Verification items for the finished model (mm, model axes). Face numbers are marked on the shaded views. A direction names the side the tool comes from. Coordinates: 2 decimals unless noted, no trailing zeros. Write each loop counter-clockwise with the first axis right and the second up, starting at its lowest first coordinate (ties: lowest second). Pieces come first, ordered by that corner, then holes.
```python
from build123d import *

# Parameters (mm, degrees)
SKETCH1_R           = 6
SKETCH1_R_2         = 1.5
BOSS_EXTRUDE1_DEPTH = 59
SKETCH2_W           = 49
SKETCH2_H           = 46
CUT_EXTRUDE1_DEPTH  = 291.342900723
SKETCH3_W           = 9
SKETCH3_H           = 50
SKETCH3_W_2         = 22
SKETCH3_W_3         = 19
CUT_EXTRUDE2_DEPTH  = 290.584184651
CUT_EXTRUDE3_DEPTH  = 4
SKETCH7_R           = 2.55
CUT_EXTRUDE4_DEPTH  = 82
CUT_EXTRUDE5_DEPTH  = 4
SKETCH9_R           = 1.5
CUT_EXTRUDE6_DEPTH  = 290.584184651


with BuildPart() as part:
    # Sketch1 → Boss-Extrude1 (new body)
    with BuildSketch(Plane(origin=(0, 0, 0), x_dir=(0, 0, -1), z_dir=(1, 0, 0))):
        with BuildLine():
            Line((3, 15), (3, 0))
            Line((3, 0), (283, 0))
            Line((283, 0), (283, 23))
            Line((283, 23), (235, 23))
            Line((235, 23), (235, 10))
            Line((235, 10), (197, 10))
            ThreePointArc((197, 10), (187.807611845, 13.807611845), (184, 23))
            ThreePointArc((184, 23), (180, 27), (176, 23))
            ThreePointArc((176, 23), (172.192388155, 13.807611845), (163, 10))
            Line((163, 10), (32, 10))
            ThreePointArc((32, 10), (28.464466094, 11.464466094), (27, 15))
            ThreePointArc((27, 15), (23.485281374, 23.485281374), (15, 27))
            ThreePointArc((15, 27), (6.514718626, 23.485281374), (3, 15))
        make_face()
        with Locations((15, 15)):
            Circle(SKETCH1_R, mode=Mode.SUBTRACT)
        with Locations((180, 23)):
            Circle(SKETCH1_R_2, mode=Mode.SUBTRACT)
    extrude(amount=BOSS_EXTRUDE1_DEPTH)

    # Sketch2 → Cut-Extrude1 (cut, through all)
    with BuildSketch(Plane.XZ):
        with Locations((24.5, -26)):
            Rectangle(SKETCH2_W, SKETCH2_H)
    extrude(amount=-CUT_EXTRUDE1_DEPTH, mode=Mode.SUBTRACT)

    # Sketch3 → Cut-Extrude2 (cut, through all)
    with BuildSketch(Plane(origin=(0, 10, 0), x_dir=(1, 0, 0), z_dir=(0, 1, 0))):
        with Locations((31, 172)):
            Rectangle(SKETCH3_W, SKETCH3_H)
        with Locations((11, 172)):
            Rectangle(SKETCH3_W_2, SKETCH3_H)
        with Locations((49.5, 172)):
            Rectangle(SKETCH3_W_3, SKETCH3_H)
    extrude(amount=CUT_EXTRUDE2_DEPTH, mode=Mode.SUBTRACT)

    # Sketch6 → Cut-Extrude3 (cut)
    with BuildSketch(Plane(origin=(0, 0, -283), x_dir=(-1, 0, 0), z_dir=(0, 0, -1))):
        Polygon((-49, 10.381197846), (-45, 12.690598923), (-45, 17.309401077), (-49, 19.618802154), (-53, 17.309401077), (-53, 12.690598923), align=None)
        Polygon((-9, 10.381197846), (-5, 12.690598923), (-5, 17.309401077), (-9, 19.618802154), (-13, 17.309401077), (-13, 12.690598923), align=None)
    extrude(amount=-CUT_EXTRUDE3_DEPTH, mode=Mode.SUBTRACT)

    # Sketch7 → Cut-Extrude4 (cut)
    with BuildSketch(Plane(origin=(0, 0, -279), x_dir=(-1, 0, 0), z_dir=(0, 0, -1))):
        with Locations((-49, 15)):
            Circle(SKETCH7_R)
        with Locations((-9, 15)):
            Circle(SKETCH7_R)
    extrude(amount=-CUT_EXTRUDE4_DEPTH, mode=Mode.SUBTRACT)

    # Sketch8 → Cut-Extrude5 (cut)
    with BuildSketch(Plane.XY.offset(-235)):
        Polygon((9, 10.381197846), (13, 12.690598923), (13, 17.309401077), (9, 19.618802154), (5, 17.309401077), (5, 12.690598923), align=None)
        Polygon((49, 10.381197846), (53, 12.690598923), (53, 17.309401077), (49, 19.618802154), (45, 17.309401077), (45, 12.690598923), align=None)
    extrude(amount=-CUT_EXTRUDE5_DEPTH, mode=Mode.SUBTRACT)

    # Sketch9 → Cut-Extrude6 (cut, through all)
    with BuildSketch(Plane(origin=(0, 10, 0), x_dir=(1, 0, 0), z_dir=(0, 1, 0))):
        with Locations(Location((27.75, 71.5, 0), (0, 0, 270))):
            Circle(SKETCH9_R)
        with Locations(Location((27.75, 85.74, 0), (0, 0, 270))):
            Circle(SKETCH9_R)
        with Locations(Location((27.75, 101.6, 0), (0, 0, 270))):
            Circle(SKETCH9_R)
        with Locations(Location((27.75, 116.72, 0), (0, 0, 270))):
            Circle(SKETCH9_R)
        with Locations(Location((32.75, 187.78, 0), (0, 0, 270))):
            Circle(SKETCH9_R)
        with Locations(Location((32.75, 214.06, 0), (0, 0, 270))):
            Circle(SKETCH9_R)
    extrude(amount=-CUT_EXTRUDE6_DEPTH, mode=Mode.SUBTRACT)


solid = part.part
```
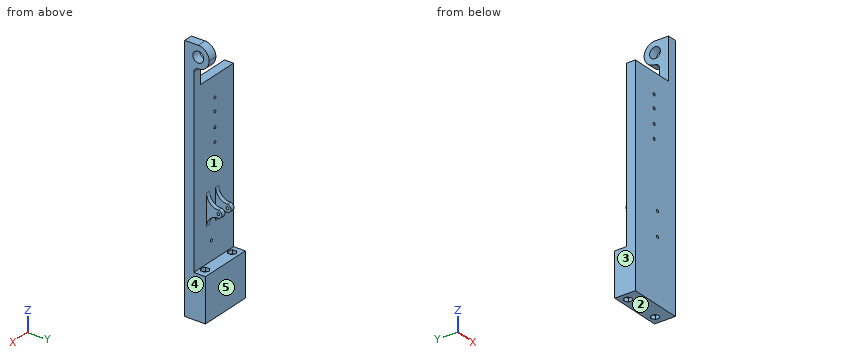
1. Sectioned sample at A-A, the plane z = -139. Record the boundary of the cut face in (x, y), and give its area (3 significant figures).
2. Gauge pin test, flat ends, axial feed: P1, Ø4, axis at y = 23, z = -180, coming from the +X side; P2, Ø13.5, axis at y = 21, z = -173, coming from the -X side; P3, Ø8, axis at y = 15, z = -25, coming from the -X side. Record the tip position at first contact, or that the pin passes through.
3. Draft check along Z on the marked faces 1, 2 and 3. Enter one of: pulls with the +Z half, pulls with the -Z half, needs draft (parallel to the pull), parting line crosses it, or undercut.
4. Tool access check on the marked faces 4 and 5. Record the directions out of +Z, -Z, +X, -X, +Y, -Y that give a thin tool (end or side, any length) a straight path to the whole face; none if there is none.
5. Material ranges on L1, parallel to X at y = 2.75, z = -101.6; L2, parallel to X at y = 2.75, z = -214.06; L3, parallel to Y at x = 24, z = -180, recorded low to high.
Outcome:
1. outline: (0, 0) - (59, 0) - (59, 10) - (0, 10) - close
1. area: 590 mm2
2. P1: stops at x = 40
2. P2: stops at x = 22
2. P3: stops at x = 49
3. face 1: undercut
3. face 2: pulls with the -Z half
3. face 3: needs draft
4. face 4: +Z, -Z, +X, +Y, -Y
4. face 5: -Z, +X, -X, +Y
5. L1: x = 0 to 26.25, 29.25 to 59
5. L2: x = 0 to 31.25, 34.25 to 59
5. L3: y = 0 to 21.5, 24.5 to 27
